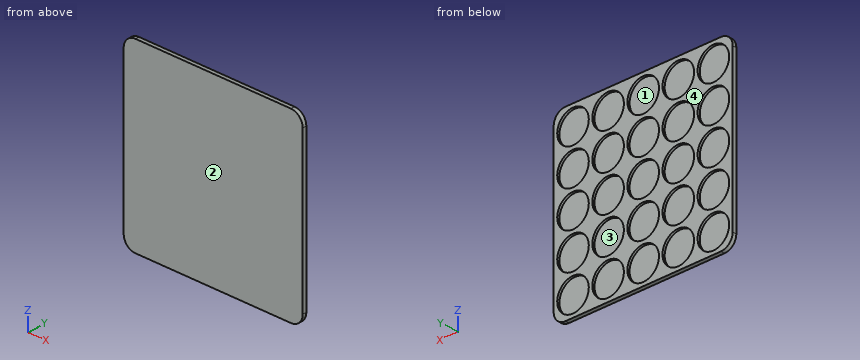
```python
from build123d import *

# Parameters (mm, degrees)
SKETCH1_W           = 229.5
SKETCH1_H           = 229.5
BOSS_EXTRUDE1_DEPTH = 5
SKETCH2_R           = 20.25
CUT_EXTRUDE1_DEPTH  = 3
FILLET1_R           = 15


with BuildPart() as part:
    # Sketch1 → Boss-Extrude1 (new body)
    with BuildSketch(Plane(origin=(0, 0, 0), x_dir=(1, 0, 0), z_dir=(0, 1, 0))):
        Rectangle(SKETCH1_W, SKETCH1_H)
    extrude(amount=BOSS_EXTRUDE1_DEPTH)

    # Sketch2 → Cut-Extrude1 (cut)
    with BuildSketch(Plane(origin=(0, 5, 0), x_dir=(1, 0, 0), z_dir=(0, 1, 0))):
        with Locations(Location((-90, 90, 0), (0, 0, 270))):
            Circle(SKETCH2_R)
        with Locations(Location((-45, 90, 0), (0, 0, 270))):
            Circle(SKETCH2_R)
        with Locations(Location((0, 90, 0), (0, 0, 270))):
            Circle(SKETCH2_R)
        with Locations(Location((45, 90, 0), (0, 0, 270))):
            Circle(SKETCH2_R)
        with Locations(Location((90, 90, 0), (0, 0, 270))):
            Circle(SKETCH2_R)
        with Locations(Location((-45, 45, 0), (0, 0, 270))):
            Circle(SKETCH2_R)
        with Locations(Location((0, 45, 0), (0, 0, 270))):
            Circle(SKETCH2_R)
        with Locations(Location((45, 45, 0), (0, 0, 270))):
            Circle(SKETCH2_R)
        with Locations(Location((90, 45, 0), (0, 0, 270))):
            Circle(SKETCH2_R)
        with Locations(Location((-45, 0, 0), (0, 0, 270))):
            Circle(SKETCH2_R)
        with Locations(Location((0, 0, 0), (0, 0, 270))):
            Circle(SKETCH2_R)
        with Locations(Location((45, 0, 0), (0, 0, 270))):
            Circle(SKETCH2_R)
        with Locations(Location((90, 0, 0), (0, 0, 270))):
            Circle(SKETCH2_R)
        with Locations(Location((-45, -45, 0), (0, 0, 270))):
            Circle(SKETCH2_R)
        with Locations(Location((0, -45, 0), (0, 0, 270))):
            Circle(SKETCH2_R)
        with Locations(Location((45, -45, 0), (0, 0, 270))):
            Circle(SKETCH2_R)
        with Locations(Location((90, -45, 0), (0, 0, 270))):
            Circle(SKETCH2_R)
        with Locations(Location((-45, -90, 0), (0, 0, 270))):
            Circle(SKETCH2_R)
        with Locations(Location((0, -90, 0), (0, 0, 270))):
            Circle(SKETCH2_R)
        with Locations(Location((45, -90, 0), (0, 0, 270))):
            Circle(SKETCH2_R)
        with Locations(Location((90, -90, 0), (0, 0, 270))):
            Circle(SKETCH2_R)
        with Locations(Location((-90, 45, 0), (0, 0, 270))):
            Circle(SKETCH2_R)
        with Locations(Location((-90, 0, 0), (0, 0, 270))):
            Circle(SKETCH2_R)
        with Locations(Location((-90, -45, 0), (0, 0, 270))):
            Circle(SKETCH2_R)
        with Locations(Location((-90, -90, 0), (0, 0, 270))):
            Circle(SKETCH2_R)
    extrude(amount=-CUT_EXTRUDE1_DEPTH, mode=Mode.SUBTRACT)

    # Fillet1
    fillet1_edges = [part.edges().sort_by_distance(p)[0] for p in [
        (114.75, 2.5, 114.75),
        (-114.75, 2.5, 114.75),
        (-114.75, 2.5, -114.75),
        (114.75, 2.5, -114.75),
    ]]
    fillet(fillet1_edges, radius=FILLET1_R)


solid = part.part
```
Source: CAD feature listing. Evaluate the final solid. Frame: model axes, mm. Face numbers are marked on the shaded views. A direction names the side the tool comes from. Give positions to 0.01 mm unless a question says otherwise; leave off trailing zeros. Loops run counter-clockwise (first coordinate to the right, second up) from the corner with the lowest first, then second, coordinate; pieces in that order, holes last. Notation, with made-up numbers: (68.25, 22) -> (100.25, 22) arc R32 cw to (100.25, 58) -> close; hole circle Ø6 at (-10, 19.25). An arc over 180 degrees is marked (long way). Use a Markdown table: item, result. Add a question column.
(1) Section query A-A (x = -45). Output: boundary loops of the cut face in (y, z).
(2) Access query for the marked faces 1 and 2. Directions: +Z, -Z, +X, -X, +Y, -Y. A direction counts if a zero-diameter tool reaches every point of the face in a straight line with its end or side. Return the directions, or none.
(3) Ray query, line 1 (X direction, y = 4.1, z = -90); line 2 (X direction, y = 4.3, z = 7.5); line 3 (Z direction, x = -76.5, y = 4.7). Return the intervals inside material, ascending.
(4) Pull-direction query (Z, two-part tool) for the marked faces 3 and 4; classes: +Z half, -Z half, draft (parallel to the pull), parting line (faces both ways), or undercut.
(5) Section query B-B (z = 45). Output: boundary loops of the cut face in (x, y).
(6) First-contact query: pin 1 Ø20 at (x, z) = (43.5, -8.5) entering from +Y. Flat tip, straight axial feed; report the tip coordinate or a pass-through.
Checked values:
| question | item | result |
|---|---|---|
| 1 | outline | (0, -114.75) -> (5, -114.75) -> (5, -110.25) -> (2, -110.25) -> (2, -69.75) -> (5, -69.75) -> (5, -65.25) -> (2, -65.25) -> (2, -24.75) -> (5, -24.75) -> (5, -20.25) -> (2, -20.25) -> (2, 20.25) -> (5, 20.25) -> (5, 24.75) -> (2, 24.75) -> (2, 65.25) -> (5, 65.25) -> (5, 69.75) -> (2, 69.75) -> (2, 110.25) -> (5, 110.25) -> (5, 114.75) -> (0, 114.75) -> close |
| 2 | face 1 | +Y |
| 2 | face 2 | +Z, -Z, +X, -X, -Y |
| 3 | line 1 | -114.75 to -110.25, -69.75 to -65.25, -24.75 to -20.25, 20.25 to 24.75, 65.25 to 69.75, 110.25 to 114.75 |
| 3 | line 2 | -114.75 to -108.81, -71.19 to -63.81, -26.19 to -18.81, 18.81 to 26.19, 63.81 to 71.19, 108.81 to 114.75 |
| 3 | line 3 | -114.75 to -105.09, -74.91 to -60.09, -29.91 to -15.09, 15.09 to 29.91, 60.09 to 74.91, 105.09 to 114.75 |
| 4 | face 3 | undercut |
| 4 | face 4 | draft |
| 5 | outline | (-114.75, 0) -> (114.75, 0) -> (114.75, 5) -> (110.25, 5) -> (110.25, 2) -> (69.75, 2) -> (69.75, 5) -> (65.25, 5) -> (65.25, 2) -> (24.75, 2) -> (24.75, 5) -> (20.25, 5) -> (20.25, 2) -> (-20.25, 2) -> (-20.25, 5) -> (-24.75, 5) -> (-24.75, 2) -> (-65.25, 2) -> (-65.25, 5) -> (-69.75, 5) -> (-69.75, 2) -> (-110.25, 2) -> (-110.25, 5) -> (-114.75, 5) -> close |
| 6 | pin 1 | y = 2 |
